Source: CAD feature listing. Evaluate the final solid. Frame: model axes, mm. A direction names the side the tool comes from. Round coordinates to 2 decimals unless told otherwise and drop trailing zeros. Loops run counter-clockwise (first coordinate to the right, second up) from the corner with the lowest first, then second, coordinate; pieces in that order, holes last. Notation, with made-up numbers: M 72.5,-32 L 105.5,-32 A29 ccw 105.5,-2 Z; hole C -35,41.5 d1. An arc over 180 degrees is marked long. One line per item, written item: value.
from build123d import *

# Parameters (mm, degrees)
CROQUIS1_R              = 10
SALIENTE_EXTRUIR1_DEPTH = 100
CROQUIS2_R              = 10
CROQUIS2_R_2            = 2.75
SALIENTE_EXTRUIR2_DEPTH = 3
CROQUIS3_R              = 0.9
CORTAR_EXTRUIR1_DEPTH   = 10


with BuildPart() as part:
    # Croquis1 → Saliente-Extruir1 (new body)
    with BuildSketch(Plane.XZ.offset(56.611885127)):
        with Locations((-3.039414363, 30.619510909)):
            Circle(CROQUIS1_R)
        with BuildLine():
            Line((-1.039414363, 38.365477601), (-1.039414363, 34.619510909))
            Line((-1.039414363, 34.619510909), (-5.039414363, 34.619510909))
            Line((-5.039414363, 34.619510909), (-5.039414363, 38.365477601))
            ThreePointArc((-5.039414363, 38.365477601), (-3.039414363, 22.619510909), (-1.039414363, 38.365477601))
        make_face(mode=Mode.SUBTRACT)
    extrude(amount=SALIENTE_EXTRUIR1_DEPTH)

    # Croquis2 → Saliente-Extruir2 (add)
    with BuildSketch(Plane.XZ.offset(156.611885127)):
        with Locations((-3.039414363, 30.619510909)):
            Circle(CROQUIS2_R)
        with Locations((-3.039414363, 30.619510909)):
            Circle(CROQUIS2_R_2, mode=Mode.SUBTRACT)
    extrude(amount=-SALIENTE_EXTRUIR2_DEPTH)

    # Croquis3 → Cortar-Extruir1 (cut)
    with BuildSketch(Plane.XZ.offset(156.611885127)):
        with Locations((-3.039414363, 37.577400418)):
            Circle(CROQUIS3_R)
        with Locations((3.918475146, 30.619510909)):
            Circle(CROQUIS3_R)
        with Locations((-3.039414363, 23.6616214)):
            Circle(CROQUIS3_R)
        with Locations((-9.997303872, 30.619510909)):
            Circle(CROQUIS3_R)
    extrude(amount=-CORTAR_EXTRUIR1_DEPTH, mode=Mode.SUBTRACT)


solid = part.part
1. Pull-direction query (Z, two-part tool) for faces 1 (the face through (-3.23, -155.13, 22.78)), 2 (the face through (3.72, -155.13, 29.74)), 3 (the face through (-3, -56.612, 35)), 4 (the face through (-5.207, -105.912, 20.857)); classes: released by +Z, released by -Z, zero draft, split by the parting line, or undercut.
Report:
face 1: undercut
face 2: undercut
face 3: zero draft
face 4: split by the parting line
2. Section query C-C (x = -7). Return the cut outline in (y, z).
Report:
outline: M -156.61,21.44 L -56.61,21.44 L -56.61,23.67 L -153.61,23.67 L -153.61,37.57 L -56.61,37.57 L -56.61,39.8 L -156.61,39.8 Z
3. Section query B-B (y = -91). Return the cut outline in (x, z).
Report:
outline: C -3.04,30.62 d20; hole M -5.04,34.62 L -5.04,38.37 A8 ccw long -1.04,38.37 L -1.04,34.62 Z
4. Pin query (flat end, axial travel): pin 1 (6.5 mm diameter, centred on x = -3.04, z = 30.62, fed in from +Y); pin 2 (1.5 mm diameter, centred on y = -112, z = 27, fed in from -X); pin 3 (3 mm diameter, centred on x = -7.5, y = -73, fed in from +Z). Return the tip coordinate at first contact, or that it passes through.
Report:
pin 1: stops at y = -153.61
pin 2: stops at x = -12.62
pin 3: stops at z = 40.17
5. Reachability of faces 5 (the face through (-3.636, -155.133, 27.935)), 6 (the face through (-5.039, -104, 36)), 7 (the face through (-3.16, -151.68, 38.47)) from +Z, -Z, +X, -X, +Y, -Y: full face, straight path, thin tool, end or side. Return the list, or none.
Report:
face 5: +Y, -Y
face 6: +Y
face 7: -Y
6. Section query A-A (y = -150). Return the cut outline in (x, z), and give its area (3 significant figures).
Report:
outline: C -3.04,30.62 d20; hole M -5.04,34.62 L -5.04,38.37 A8 ccw long -1.04,38.37 L -1.04,34.62 Z; hole C -3.04,37.58 d1.8
area: 126 mm2
7. Ray query, line 1 (Z direction, x = -3.25, y = -74.5); line 2 (X direction, y = -87.5, z = 37.75); line 3 (Z direction, x = 1.75, y = -80). Return the intervals inside material, ascending. Write a range as [from, to].
Report:
line 1: z = [20.62, 22.62], [34.62, 40.62]
line 2: x = [-10.05, -6.67], [-5.04, -1.04], [0.59, 3.97]
line 3: z = [21.84, 24.21], [37.03, 39.4]
